```python
from build123d import *

# Parameters (mm, degrees)
F1_DEPTH = 1


with BuildPart() as f1:
    # F0 (on Top) → F1 (new body)
    with BuildSketch(Plane.XY):
        Polygon((-2, 0), (0, 0), (0, 7.5), (-20.25, 7.5), (-20.25, 4.25), (-2, 4.25), align=None)
        Polygon((3.030825, 0), (0, 0), (-2, 0), (-2, -2.433287), (5.030825, -2.433287), (5.030825, 0), align=None)
        Polygon((3.030825, 7.5), (3.030825, 0), (5.030825, 0), (5.030825, 4.25), (23.280825, 4.25), (23.280825, 7.5), align=None)
    extrude(amount=F1_DEPTH)


solid = f1.part
```
Source: CAD feature listing. Evaluate the final solid. Frame: model axes, mm. A direction names the side the tool comes from. Give positions to 0.01 mm unless a question says otherwise; leave off trailing zeros. Write each loop counter-clockwise with the first axis right and the second up, starting at its lowest first coordinate (ties: lowest second). Pieces come first, ordered by that corner, then holes.
1. Pull-direction query (X, two-part tool) for faces 1 (the face through (5.031, 0.9, 0.5)), 2 (the face through (-10, 7.5, 0.5)), 3 (the face through (3.031, 3.8, 0.5)), 4 (the face through (-20.25, 5.9, 0.5)); classes: +X half, -X half, draft (parallel to the pull), parting line (faces both ways), or undercut.
2. Access query for faces 5 (the face through (-2, 1, 0.5)), 6 (the face through (0, 3.7, 0.5)), 7 (the face through (14, 4.25, 0.5)). Directions: +Z, -Z, +X, -X, +Y, -Y. A direction counts if a zero-diameter tool reaches every point of the face in a straight line with its end or side. Return the directions, or none.
3. Section query A-A (y = 3.25). Return the cut outline in (x, z).
4. Material intervals for line 1 along X through (y, z) = (1, 0.95); line 2 along X through (y, z) = (7.25, 0.25); line 3 along Y through (x, z) = (9, 0.25), sorted ascending.
5. First-contact query: pin 1 (0.5 mm diameter, centred on x = 2.5, z = 0.5, fed in from +Y); pin 2 (0.5 mm diameter, centred on x = 10.5, z = 0.5, fed in from -Y); pin 3 (0.5 mm diameter, centred on y = 2.5, z = 0.5, fed in from +X). Flat tips, straight axial feed; report the tip coordinate or a pass-through.
6. Section query D-D (x = 0.5). Return the cut outline in (y, z).
7. Section query B-B (z = 0.2). Return the cut outline in (x, y).
8. Section query C-C (y = -1.5). Return the cut outline in (x, z), then the cut area to 3 significant figures.
Output values:
1. face 1: +X half
1. face 2: draft
1. face 3: undercut
1. face 4: -X half
2. face 5: +Z, -Z, -X, -Y
2. face 6: +Z, -Z, +Y
2. face 7: +Z, -Z, +X, -Y
3. outline: (-2, 0) - (0, 0) - (0, 1) - (-2, 1) - close; (3.03, 0) - (5.03, 0) - (5.03, 1) - (3.03, 1) - close
4. line 1: x = -2 to 0, 3.03 to 5.03
4. line 2: x = -20.25 to 0, 3.03 to 23.28
4. line 3: y = 4.25 to 7.5
5. pin 1: stops at y = 0
5. pin 2: stops at y = 4.25
5. pin 3: stops at x = 5.03
6. outline: (-2.43, 0) - (0, 0) - (0, 1) - (-2.43, 1) - close
7. outline: (-20.25, 4.25) - (-2, 4.25) - (-2, -2.43) - (5.03, -2.43) - (5.03, 4.25) - (23.28, 4.25) - (23.28, 7.5) - (3.03, 7.5) - (3.03, 0) - (0, 0) - (0, 7.5) - (-20.25, 7.5) - close
8. outline: (-2, 0) - (5.03, 0) - (5.03, 1) - (-2, 1) - close
8. area: 7.03 mm2
